```python
from build123d import *

# Parameters (mm, degrees)
F0_R     = 12.7
F1_DEPTH = 2.54
F2_R     = 0.635
F3_DEPTH = 25.4
F4_R     = 1.26999


# Not quite as in the source:
# - a fillet or chamfer is up to 0.001 mm smaller than in the source, because OpenCascade refuses the exact size


with BuildPart() as f1:
    # F0 (on Front) → F1 (new body)
    with BuildSketch(Plane.XZ):
        Circle(F0_R)
    extrude(amount=F1_DEPTH)

    # F2 (on face) → F3 (cut)
    with BuildSketch(Plane.XZ.offset(2.54)):
        Circle(F2_R)
    extrude(amount=-F3_DEPTH, mode=Mode.SUBTRACT)

    # F4 (radius 1.27 in the source; OpenCascade refuses exactly that, so slightly less here)
    f4_edges = [f1.edges().sort_by_distance(p)[0] for p in [
        (-12.7, -2.54, 0),
        (-12.7, 0, 0),
    ]]
    fillet(f4_edges, radius=F4_R)


solid = f1.part
```
Design review of the part built by this model. Coordinates are the model's own, in mm. Coordinates: 2 decimals unless noted, no trailing zeros. Loops run counter-clockwise (first coordinate to the right, second up) from the corner with the lowest first, then second, coordinate; pieces in that order, holes last.
Q1. The part is to be moulded in two halves that separate along Z. For faces 1 (the face through (0, -2.54, -2)), 2 (the face through (-0.08, -1.29, 0.63)), say which applies: +Z half, -Z half, draft (parallel to the pull), parting line (faces both ways), or undercut.
Reported:
face 1: draft
face 2: undercut
Q2. To check wall thickness, follow line 1 (Z direction, x = 0, y = -1.15) (3 decimals); line 2 (Z direction, x = 0, y = -0.75) (3 decimals); line 3 (X direction, y = -0.75, z = 1.25). State the ranges of each line that lie inside material, in increasing order.
Reported:
line 1: z = -12.694 to -0.635, 0.635 to 12.694
line 2: z = -12.589 to -0.635, 0.635 to 12.589
line 3: x = -12.53 to 12.53
Q3. We need section D-D on y = -0.4. State the section outline as (x, z) points (3 decimals), and give its area (3 significant figures).
Reported:
outline: circle Ø24.71 at (0, 0); hole circle Ø1.27 at (0, 0)
area: 478 mm2
Q4. We need section C-C on y = -1.95. State the section outline as (x, z) points (3 decimals), and give its area (3 significant figures).
Reported:
outline: circle Ø25.005 at (0, 0); hole circle Ø1.27 at (0, 0)
area: 490 mm2
